Autodesk Inventor part; units mm, degrees
ref_plane "YZ Plane" through (0, 0, 0) normal (1, 0, 0) x (0, 1, 0)
ref_plane "XZ Plane" through (0, 0, 0) normal (0, 1, 0) x (-1, 0, 0)
ref_plane "XY Plane" through (0, 0, 0) normal (0, 0, 1) x (1, 0, 0)
sketch "Skizze1" plane through (0, 0, 0) normal (0, 0, 1) x (1, 0, 0)
  line L0 (0, 0) -> (0, 16.3048)
  line L1 (0, 0) -> (14.75, 0)
  line L2 (14.75, 0) -> (15.5, 1)
  line L3 (15.5, 1) -> (0, 1)
  dimension "d1" = 31
  dimension "d2" = 29.5
  dimension "d3" = 1
revolve "Umdrehung1" add sketch "Skizze1" angle 360 about axis through (0, 0, 0) along (0, 1, 0)
shell "Wandung1" thickness 0.5 outward yes removed faces 1 at (2.935, 1, -4.2521)
sketch "Skizze2" plane through (0, 0, 0) normal (0, 1, 0) x (1, 0, 0)
  circle A0 centre (0, 0) radius 0.81
  dimension "d5" = 1.62
extrude "Extrusion1" cut sketch "Skizze2" against normal up to surface (0.5 mm away)
properties part number "mesh filter"
Model file for the job. Use its own axes, mm. Round coordinates to 2 decimals unless told otherwise and drop trailing zeros. Order: outer loops, then holes, each group sorted by start corner. A loop starts at its lowest first (then second) coordinate and runs counter-clockwise, first axis right, second up.
(1) Band-saw the part on A-A (x = 0). List the corners of the cut face in (y, z) (3 decimals), then the cut area to 3 significant figures.
(2) Pin check, flat tips, straight feed: pin 1 (1 mm diameter, centred on x = -3, z = -12.5, fed in from +Y); pin 2 (15 mm diameter, centred on x = -6, z = -5, fed in from +Y). Stop position of each tip, or through.
(3) Drill centre lines: line 1 (X direction, y = -0.2, z = 0) (3 decimals); line 2 (Z direction, x = -7.5, y = 0.65); line 3 (Y direction, x = 7.5, z = 10.5). Where is each one in solid material? Low to high.
(4) Pull direction X, two halves, no side cores. Call faces 1 (the face through (-8.44, 1, -13.21)), 2 (the face through (0, 0, 3)): released by +X, released by -X, zero draft, split by the parting line, or undercut.
(5) Band-saw the part on C-C (y = 0.55). List the corners of the cut face in (x, z) (1 decimal), then the cut area to 3 significant figures.
(6) Band-saw the part on B-B (z = 0). List the corners of the cut face in (x, y) (3 decimals).
Verdict:
1. outline: (-0.5, -15) - (1, -16.125) - (1, -15.5) - (0, -14.75) - (0, -0.81) - (-0.5, -0.81) - close; (-0.5, 0.81) - (0, 0.81) - (0, 14.75) - (1, 15.5) - (1, 16.125) - (-0.5, 15) - close
1. area: 15.6 mm2
2. pin 1: stops at y = 0
2. pin 2: stops at y = 0.75
3. line 1: x = -15.225 to -0.81, 0.81 to 15.225
3. line 2: z = -13.98 to -13.26, 13.26 to 13.98
3. line 3: y = -0.5 to 0
4. face 1: zero draft
4. face 2: undercut
5. outline: circle Ø31.6 at (0, 0); hole circle Ø30.3 at (0, 0)
5. area: 60.8 mm2
6. outline: (-16.125, 1) - (-15, -0.5) - (-0.81, -0.5) - (-0.81, 0) - (-14.75, 0) - (-15.5, 1) - close; (0.81, -0.5) - (15, -0.5) - (16.125, 1) - (15.5, 1) - (14.75, 0) - (0.81, 0) - close
